Part model, mm, in its own coordinate system. Give positions to 0.01 mm unless a question says otherwise; leave off trailing zeros. Write each loop counter-clockwise with the first axis right and the second up, starting at its lowest first coordinate (ties: lowest second). Pieces come first, ordered by that corner, then holes.
from build123d import *

# Parameters (mm, degrees)
F1_DEPTH = 6.35


with BuildPart() as f1:
    # F0 (on Top) → F1 (new body)
    with BuildSketch(Plane.XY):
        with BuildLine():
            ThreePointArc((-30.0819607702, 11.9151759356), (-20.3578704511, 13.8767489709), (-13.1982271915, 20.7429859098))
            ThreePointArc((-13.1982271915, 20.7429859098), (-11.4219976513, 25.0311833169), (-10.816158833, 29.6329859753))
            ThreePointArc((-10.816158833, 29.6329859753), (-11.179762963, 33.2103530099), (-12.2557038161, 36.6414044732))
            ThreePointArc((-12.2557038161, 36.6414044732), (-43.0187721174, 40.03090048), (-30.0819607702, 11.9151759356))
        make_face()
        with BuildLine():
            ThreePointArc((-17.547158833, 29.6329859753), (-17.9236443783, 26.773294346), (-19.0274441465, 24.1084859753))
            ThreePointArc((-19.0274441465, 24.1084859753), (-39.2686732876, 32.4926776046), (-17.547158833, 29.6329859753))
        make_face(mode=Mode.SUBTRACT)
        with BuildLine():
            ThreePointArc((13.6786666056, 39.3075312177), (10.8221098654, 30.0929678224), (13.1982271824, 20.7429859256))
            ThreePointArc((13.1982271824, 20.7429859256), (20.7152486277, 13.6949919254), (30.8792758859, 12.0001819861))
            ThreePointArc((30.8792758859, 12.0001819861), (41.9513492322, 17.8955548509), (46.376158833, 29.6329859753))
            ThreePointArc((46.376158833, 29.6329859753), (33.6407295877, 46.6823468402), (13.6786666056, 39.3075312177))
        make_face()
        with BuildLine():
            ThreePointArc((39.645158833, 29.6329859753), (31.4558504623, 18.9604715206), (19.0274441465, 24.1084859753))
            ThreePointArc((19.0274441465, 24.1084859753), (25.7364672036, 40.30550043), (39.645158833, 29.6329859753))
        make_face(mode=Mode.SUBTRACT)
        with BuildLine():
            ThreePointArc((14.9259864768, -10.2355789505), (8.4955307169, -4.2779757112), (-3.9e-09, -2.1170140247))
            ThreePointArc((-3.9e-09, -2.1170140247), (-9.5695821881, -4.9119715908), (-16.1305506354, -12.4181279982))
            ThreePointArc((-16.1305506354, -12.4181279982), (-3.8293086649, -37.259755604), (17.78, -19.8970140247))
            ThreePointArc((17.78, -19.8970140247), (17.0515752873, -14.8599334991), (14.9259864768, -10.2355789505))
        make_face()
        with BuildLine():
            ThreePointArc((11.049, -19.8970140247), (-7.8128228253, -27.70983685), (0, -8.8480140247))
            ThreePointArc((0, -8.8480140247), (7.8128228253, -12.0841911994), (11.049, -19.8970140247))
        make_face(mode=Mode.SUBTRACT)
        with BuildLine():
            ThreePointArc((30.8792758859, 12.0001819861), (20.7152486277, 13.6949919254), (13.1982271824, 20.7429859256))
            ThreePointArc((13.1982271824, 20.7429859256), (14.7207096001, 17.0673881949), (15.24, 13.1229859753))
            ThreePointArc((15.24, 13.1229859753), (10.7763073439, 2.3466786287), (-3.9e-09, -2.1170140247))
            ThreePointArc((-3.9e-09, -2.1170140247), (8.4955307169, -4.2779757112), (14.9259864768, -10.2355789505))
            ThreePointArc((14.9259864768, -10.2355789505), (18.7381800343, 3.8701324523), (30.8792758859, 12.0001819861))
        make_face()
        with BuildLine():
            ThreePointArc((-13.1982271915, 20.7429859098), (-9.1e-09, 28.3629859753), (13.1982271824, 20.7429859256))
            ThreePointArc((13.1982271824, 20.7429859256), (10.8221098654, 30.0929678224), (13.6786666056, 39.3075312177))
            ThreePointArc((13.6786666056, 39.3075312177), (1.1802177429, 33.4149013853), (-12.2557038161, 36.6414044732))
            ThreePointArc((-12.2557038161, 36.6414044732), (-11.179762963, 33.2103530099), (-10.816158833, 29.6329859753))
            ThreePointArc((-10.816158833, 29.6329859753), (-11.4219976513, 25.0311833169), (-13.1982271915, 20.7429859098))
        make_face()
        with BuildLine():
            ThreePointArc((-16.1305506354, -12.4181279982), (-9.5695821881, -4.9119715908), (-3.9e-09, -2.1170140247))
            ThreePointArc((-3.9e-09, -2.1170140247), (-13.1982271357, 5.5029859442), (-13.1982271915, 20.7429859098))
            ThreePointArc((-13.1982271915, 20.7429859098), (-20.3578704511, 13.8767489709), (-30.0819607702, 11.9151759356))
            ThreePointArc((-30.0819607702, 11.9151759356), (-18.3961354972, 2.4490540304), (-16.1305506354, -12.4181279982))
        make_face()
        with BuildLine():
            Line((0, -2.1170140247), (0, 0.1261395605))
            ThreePointArc((0, 0.1261395605), (-11.2555991643, 6.6245627679), (-11.2555991643, 19.6214091827))
            Line((-11.2555991643, 19.6214091827), (-13.1982271537, 20.7429859753))
            ThreePointArc((-13.1982271915, 20.7429859098), (-13.1982271357, 5.5029859442), (-3.9e-09, -2.1170140247))
        make_face()
        with BuildLine():
            ThreePointArc((-11.2555991643, 19.6214091827), (0, 26.1198323901), (11.2555991643, 19.6214091827))
            Line((11.2555991643, 19.6214091827), (13.1982271537, 20.7429859753))
            ThreePointArc((13.1982271824, 20.7429859256), (-9.1e-09, 28.3629859753), (-13.1982271915, 20.7429859098))
            Line((-13.1982271537, 20.7429859753), (-11.2555991643, 19.6214091827))
        make_face()
        with BuildLine():
            ThreePointArc((11.2555991643, 19.6214091827), (12.5539896124, 16.4868173537), (12.9968464148, 13.1229859753))
            ThreePointArc((12.9968464148, 13.1229859753), (9.190158234, 3.9328277413), (0, 0.1261395605))
            Line((0, 0.1261395605), (0, -2.1170140247))
            ThreePointArc((-3.9e-09, -2.1170140247), (10.7763073439, 2.3466786287), (15.24, 13.1229859753))
            ThreePointArc((15.24, 13.1229859753), (14.7207096001, 17.0673881949), (13.1982271824, 20.7429859256))
            Line((13.1982271537, 20.7429859753), (11.2555991643, 19.6214091827))
        make_face()
    extrude(amount=F1_DEPTH)


solid = f1.part
1) Saw through at A-A (y = 1.5). Write the cut outline in (x, z), and give its area (3 significant figures).
Check result:
outline: (-17.88, 0) - (-5.82, 0) - (-5.82, 6.35) - (-17.88, 6.35) - close; (5.82, 0) - (17.27, 0) - (17.27, 6.35) - (5.82, 6.35) - close
area: 149 mm2
2) Saw through at B-B (x = -32). Write the cut outline in (y, z), and give its area (3 significant figures).
Check result:
outline: (12.18, 0) - (19.12, 0) - (19.12, 6.35) - (12.18, 6.35) - close; (40.14, 0) - (47.08, 0) - (47.08, 6.35) - (40.14, 6.35) - close
area: 88.1 mm2
3) Saw through at C-C (z = 2). Write the cut outline in (x, y), and give its area (3 significant figures).
Check result:
outline: (-30.08, 11.92) arc R20.83 cw to (-16.13, -12.42) arc R17.78 ccw (long way) to (14.93, -10.24) arc R20.83 cw to (30.88, 12) arc R17.78 ccw (long way) to (13.68, 39.31) arc R20.83 cw to (-12.26, 36.64) arc R17.78 ccw (long way) to start; hole circle Ø22.1 at (-28.6, 29.63); hole circle Ø25.99 at (0, 13.12); hole circle Ø22.1 at (0, -19.9); hole circle Ø22.1 at (28.6, 29.63)
area: 2,590 mm2
4) Drill centre lines: L1, parallel to X at y = 21.5, z = 2; L2, parallel to X at y = 23, z = 5.25; L3, parallel to X at y = 28, z = 3.75. Where is each one in solid material? Low to high.
Check result:
L1: x = -44.41 to -36.08, -21.12 to -9.94, 9.94 to 21.12, 36.08 to 44.41
L2: x = -45.09 to -37.43, -19.76 to -8.45, 8.45 to 19.76, 37.43 to 45.09
L3: x = -46.3 to -39.52, -17.67 to 17.67, 39.52 to 46.3
5) Flat gauge pins, fed straight in: P1, Ø1, axis at x = 28, z = 4.5, coming from the +Y side; P2, Ø1, axis at y = -16, z = 0.5, coming from the +X side; P3, Ø2, axis at x = 1.5, z = 1.5, coming from the +Y side; P4, Ø1, axis at y = -27, z = 2.5, coming from the +X side. Where does each tip first touch, or does it go through?
Check result:
P1: stops at y = 47.41
P2: stops at x = 17.45
P3: stops at y = 33.59
P4: stops at x = 16.51
6) Mould opens along Y. For faces 1 (the flat face through (-11, 21, 6.35)), 2 (the cylindrical face through (-42.705, 40.453, 3.131)), 3 (the cylindrical face through (18.617, 3.7, 3.131)) say: +Y half, -Y half, draft (parallel to the pull), parting line (faces both ways), or undercut.
Check result:
face 1: draft
face 2: parting line
face 3: undercut
